Could you check a few things on this model? Use its own coordinates, in mm. A direction names the side the tool comes from. Give positions to 0.01 mm unless a question says otherwise; leave off trailing zeros. Write each loop counter-clockwise with the first axis right and the second up, starting at its lowest first coordinate (ties: lowest second). Pieces come first, ordered by that corner, then holes. Notation, with made-up numbers: (-1, -31.5) - (27, -31.5) arc R22 cw to (27, 2.5) - close; hole circle Ø4 at (60, 38). An arc over 180 degrees is marked (long way). Answer in a Markdown table with one row per item.
from build123d import *

# Parameters (mm, degrees)
FILLET_3_R          = 0.6
SKETCH_2_W          = 49
SKETCH_2_H          = 5
EXTRUDE_1_DEPTH     = 24.5
FILLET_4_R          = 4
CHAMFER_3_SIZE      = 1.5
CHAMFER_4_SIZE      = 1
SKETCH_3_R          = 3
CUT_EXTRUDE_1_DEPTH = 55.062463873
SKETCH_4_R          = 2.25
CUT_EXTRUDE_2_DEPTH = 55.062463873
SKETCH_5_R          = 2
CUT_EXTRUDE_3_DEPTH = 9
FILLET_7_R          = 0.4
CHAMFER_5_SIZE      = 0.8
CHAMFER_6_SIZE      = 0.8
CHAMFER_7_SIZE      = 0.8


# Read off the part's stored shape, not the designer's step: 旋转1
# Some blends are built 0.0001 mm under size
with BuildPart() as part:
    # 旋转1 outline → 旋转1 (revolve)
    with BuildSketch(Plane.XZ):
        Polygon((3.9, -35.644445464), (3.9, -34.544445464), (5.85, -34.544445464), (5.85, -35.644445464), (17.5, -35.644445464), (17.5, -20.144445464), (24.5, -20.144445464), (24.5, -15.144445464), (21.05, -15.144445464), (21.05, -12.944445464), (21.75, -12.944445464), (21.75, -10.144445464), (19, -10.144445464), (19, -17.144445464), (12.25, -17.144445464), (12.25, -9.044445464), (5.8, -9.044445464), (5.8, 5.855554536), (5.2, 5.855554536), (0, -13.053536373), (0, -35.644445464), align=None)
    revolve(axis=Axis((0, 0, 0), (0, 0, 1)))

    # 圆角3
    fillet_3_edges = [part.edges().sort_by_distance(p)[0] for p in [
        (-5.8, 0, 5.855554536),
    ]]
    fillet(fillet_3_edges, radius=FILLET_3_R - 0.0001)  # a hair under: the kernel refuses the full size

    # 草图2 → 凸台-拉伸1 (add, symmetric)
    with BuildSketch(Plane(origin=(0, 0, 0), x_dir=(1, 0, 0), z_dir=(0, 1, 0))):
        with Locations((0, 17.644445464)):
            Rectangle(SKETCH_2_W, SKETCH_2_H)
    extrude(amount=EXTRUDE_1_DEPTH, both=True)

    # 圆角4
    fillet_4_edges = [part.edges().sort_by_distance(p)[0] for p in [
        (24.5, -24.5, -17.644445464),
        (-24.5, 24.5, -17.644445464),
        (-24.5, -24.5, -17.644445464),
        (24.5, 24.5, -17.644445464),
    ]]
    fillet(fillet_4_edges, radius=FILLET_4_R)

    # 倒角3
    chamfer_3_edges = [part.edges().sort_by_distance(p)[0] for p in [
        (0, 24.5, -20.144445464),
        (-24.5, 0, -20.144445464),
        (24.5, 0, -20.144445464),
        (0, -24.5, -20.144445464),
        (23.328427125, 23.328427125, -20.144445464),
        (23.328427125, -23.328427125, -20.144445464),
        (-23.328427125, -23.328427125, -20.144445464),
        (-23.328427125, 23.328427125, -20.144445464),
    ]]
    chamfer(chamfer_3_edges, length=CHAMFER_3_SIZE)

    # 倒角4
    chamfer_4_edges = [part.edges().sort_by_distance(p)[0] for p in [
        (-21.75, 0, -10.144445464),
    ]]
    chamfer(chamfer_4_edges, length=CHAMFER_4_SIZE)

    # 草图3 → 切除-拉伸1 (cut, through all)
    with BuildSketch(Plane(origin=(0, 0, -35.644445464), x_dir=(-1, 0, 0), z_dir=(0, 0, -1))):
        Circle(SKETCH_3_R)
    extrude(amount=-CUT_EXTRUDE_1_DEPTH, mode=Mode.SUBTRACT)

    # 草图4 → 切除-拉伸2 (cut, through all)
    with BuildSketch(Plane(origin=(0, 0, -35.644445464), x_dir=(-1, 0, 0), z_dir=(0, 0, -1))):
        with Locations((-19.25, 18.931846081)):
            Circle(SKETCH_4_R)
        with Locations((19.25, 18.931846081)):
            Circle(SKETCH_4_R)
        with Locations((-19.25, -19.568153919)):
            Circle(SKETCH_4_R)
        with Locations((19.25, -19.568153919)):
            Circle(SKETCH_4_R)
    extrude(amount=-CUT_EXTRUDE_2_DEPTH, mode=Mode.SUBTRACT)

    # 草图5 → 切除-拉伸3 (cut)
    with BuildSketch(Plane(origin=(0, 0, -35.644445464), x_dir=(-1, 0, 0), z_dir=(0, 0, -1))):
        with Locations((-8.5, 8.5)):
            Circle(SKETCH_5_R)
        with Locations((8.5, 8.5)):
            Circle(SKETCH_5_R)
        with Locations((8.5, -8.5)):
            Circle(SKETCH_5_R)
        with Locations((-8.5, -8.5)):
            Circle(SKETCH_5_R)
    extrude(amount=-CUT_EXTRUDE_3_DEPTH, mode=Mode.SUBTRACT)

    # 圆角7
    fillet_7_edges = [part.edges().sort_by_distance(p)[0] for p in [
        (-17.5, 0, -35.644445464),
    ]]
    fillet(fillet_7_edges, radius=FILLET_7_R)

    # 倒角5
    chamfer_5_edges = [part.edges().sort_by_distance(p)[0] for p in [
        (-12.25, 0, -9.044445464),
    ]]
    chamfer(chamfer_5_edges, length=CHAMFER_5_SIZE)

    # 倒角6
    # the kernel refuses this chamfer: 0.8 mm, written as the material it takes off along each edge
    with BuildSketch(Plane(origin=(0, 0, -12.944445464), x_dir=(1, 0, 0), z_dir=(0, -1, 0))) as chamfer_6_piece_1_section:
        Polygon((21.75, CHAMFER_6_SIZE), (21.75 - CHAMFER_6_SIZE, 0), (21.75, 0), align=None)
    chamfer_6_piece_1 = revolve(axis=Axis((0, 0, -12.944445464), (0, 0, 1)), mode=Mode.PRIVATE)
    chamfer_6_piece_1 = chamfer_6_piece_1 - Plane(origin=(0, 0, -12.50853459), x_dir=(1, 0, 0), z_dir=(0, 0, 1)) * Cylinder(21.05, 87, mode=Mode.PRIVATE)
    add(chamfer_6_piece_1, mode=Mode.SUBTRACT)

    # 倒角7
    chamfer_7_edges = [part.edges().sort_by_distance(p)[0] for p in [
        (0, 24.5, -15.144445464),
        (24.5, 0, -15.144445464),
        (-24.5, 0, -15.144445464),
        (0, -24.5, -15.144445464),
        (23.328427125, 23.328427125, -15.144445464),
        (23.328427125, -23.328427125, -15.144445464),
        (-23.328427125, -23.328427125, -15.144445464),
        (-23.328427125, 23.328427125, -15.144445464),
    ]]
    chamfer(chamfer_7_edges, length=CHAMFER_7_SIZE)


solid = part.part
1) We'd pull the mould along Y, two halves only. Please class faces 5 (the face through (8.767, -16.856, -12.679)), 6 (the face through (0.287, -23.76, -19.384)), 7 (the face through (22.663, 22.712, -19.551)): +Y half, -Y half, draft (parallel to the pull), parting line (faces both ways), or undercut.
Check values:
| item | result |
|---|---|
| face 5 | undercut |
| face 6 | -Y half |
| face 7 | +Y half |
2) Imagine slicing it at A-A (z = -28). List the corners of the cut face in (x, y) for me.
Check values:
| item | result |
|---|---|
| outline | circle Ø35 at (0, 0); hole circle Ø4 at (-8.5, -8.5); hole circle Ø4 at (-8.5, 8.5); hole circle Ø6 at (0, 0); hole circle Ø4 at (8.5, -8.5); hole circle Ø4 at (8.5, 8.5) |
3) Imagine slicing it at C-C (z = -1). List the corners of the cut face in (x, y) for me, then the cut area to 3 significant figures.
Check values:
| item | result |
|---|---|
| outline | circle Ø11.6 at (0, 0); hole circle Ø6.63 at (0, 0) |
| area | 71.2 mm2 |
4) Imagine slicing it at B-B (z = -7). List the corners of the cut face in (x, y) for me.
Check values:
| item | result |
|---|---|
| outline | circle Ø11.6 at (0, 0); hole circle Ø6 at (0, 0) |
5) Will these pins go through, and if not, where does the flat tip stop? P1, Ø10, axis at x = 10.5, z = -30, coming from the -Y side; P2, Ø2, axis at x = 15.5, z = -30.5, coming from the +Y side; P3, Ø5, axis at x = 19.25, y = -19.57, coming from the +Z side.
Check values:
| item | result |
|---|---|
| P1 | stops at y = -16.61 |
| P2 | stops at y = 9.8 |
| P3 | stops at z = -15.14 |
6) If I drill on line 1 (Y direction, x = -19.25, z = -17.75); line 2 (Y direction, x = 8.5, z = -32.5); line 3 (X direction, y = 8, z = -33), over which ranges is the centre line in solid material (lowest first)?
Check values:
| item | result |
|---|---|
| line 1 | y = -24.5 to -21.82, -17.32 to 16.68, 21.18 to 24.5 |
| line 2 | y = -15.3 to -10.5, -6.5 to 6.5, 10.5 to 15.3 |
| line 3 | x = -15.56 to -10.44, -6.56 to 6.56, 10.44 to 15.56 |
7) On a 3-axis mill with a long thin cutter (end or side, diameter ignored), from which of +Z, -Z, +X, -X, +Y, -Y can I reach the whole of each face in a straight line? I mean faces 1 (the face through (3, 0, -19)), 2 (the face through (-5.794, 0.255, -1.794)), 3 (the face through (-21.4, 0.3, -15.144)), 4 (the face through (-13.887, -10.648, -27.589)). Say none if no direction works.
Check values:
| item | result |
|---|---|
| face 1 | +Z, -Z |
| face 2 | +Z |
| face 3 | none |
| face 4 | -Z |
